For this review, take the finished solid that the model builds, in its own axes (mm). Face numbers are marked on the shaded views. A direction names the side the tool comes from. Coordinates: 2 decimals unless noted, no trailing zeros. Write each loop counter-clockwise with the first axis right and the second up, starting at its lowest first coordinate (ties: lowest second). Pieces come first, ordered by that corner, then holes.
```python
from build123d import *

# Parameters (mm, degrees)
BOSS_EXTRUDE1_DEPTH     = 15.748
BOSS_EXTRUDE3_DEPTH     = 47.752
SKETCH4_W               = 31.75
SKETCH4_H               = 47.752
BOSS_EXTRUDE4_DEPTH     = 15.748
FILLET1_R               = 12.7
CUT_EXTRUDE1_DEPTH      = 133.971969005
CUT_EXTRUDE1_DEPTH_BACK = 133.971969005
SKETCH5_R               = 9.525
CUT_EXTRUDE2_DEPTH      = 132.063135736
CUT_EXTRUDE2_DEPTH_BACK = 132.063135736
SKETCH6_R               = 9.525


with BuildPart() as part:
    # Sketch1 → Boss-Extrude1 (new body)
    with BuildSketch(Plane.XY):
        with BuildLine():
            Line((-28.575, 0), (-95.292827815, 0))
            Line((-95.292827815, 0), (-95.292827815, -79.502))
            Line((-95.292827815, -79.502), (95.207172185, -79.502))
            Line((95.207172185, -79.502), (95.207172185, 0))
            Line((95.207172185, 0), (28.575, 0))
            ThreePointArc((28.575, 0), (0, -28.575), (-28.575, 0))
        make_face()
    extrude(amount=BOSS_EXTRUDE1_DEPTH)

    # Sketch2 → Boss-Extrude3 (add)
    with BuildSketch(Plane.XY.offset(15.748)):
        with BuildLine():
            Line((-44.45, 0), (-44.45, -79.502))
            Line((-44.45, -79.502), (44.45, -79.502))
            Line((44.45, -79.502), (44.45, 0))
            Line((44.45, 0), (28.575, 0))
            ThreePointArc((28.575, 0), (0, -28.575), (-28.575, 0))
            Line((-28.575, 0), (-44.45, 0))
        make_face()
    extrude(amount=BOSS_EXTRUDE3_DEPTH)

    # Sketch4 → Boss-Extrude4 (add)
    with BuildSketch(Plane.XZ.offset(79.502)):
        with Locations((-60.325, 39.624)):
            Rectangle(SKETCH4_W, SKETCH4_H)
        with Locations((60.325, 39.624)):
            Rectangle(SKETCH4_W, SKETCH4_H)
    extrude(amount=-BOSS_EXTRUDE4_DEPTH)

    # Fillet1
    fillet1_edges = [part.edges().sort_by_distance(p)[0] for p in [
        (-76.2, -71.628, 63.5),
        (76.2, -71.628, 63.5),
    ]]
    fillet(fillet1_edges, radius=FILLET1_R)

    # Sketch5 → Cut-Extrude1 (cut, two sides: drawn at the far end of the back side and taken through both)
    with BuildSketch(Plane.XY.offset(15.748).offset(-CUT_EXTRUDE1_DEPTH_BACK)):
        with Locations((63.5, -28.702)):
            Circle(SKETCH5_R)
        with Locations((-63.5, -28.702)):
            Circle(SKETCH5_R)
    extrude(amount=CUT_EXTRUDE1_DEPTH + CUT_EXTRUDE1_DEPTH_BACK, mode=Mode.SUBTRACT)

    # Sketch6 → Cut-Extrude2 (cut, two sides: drawn at the far end of the back side and taken through both)
    with BuildSketch(Plane(origin=(0, -63.754, 0), x_dir=(1, 0, 0), z_dir=(0, 1, 0)).offset(-CUT_EXTRUDE2_DEPTH_BACK)):
        with Locations(Location((-58.42, -38.1, 0), (0, 0, 270))):
            Circle(SKETCH6_R)
        with Locations(Location((58.42, -38.1, 0), (0, 0, 270))):
            Circle(SKETCH6_R)
    extrude(amount=CUT_EXTRUDE2_DEPTH + CUT_EXTRUDE2_DEPTH_BACK, mode=Mode.SUBTRACT)


solid = part.part
```
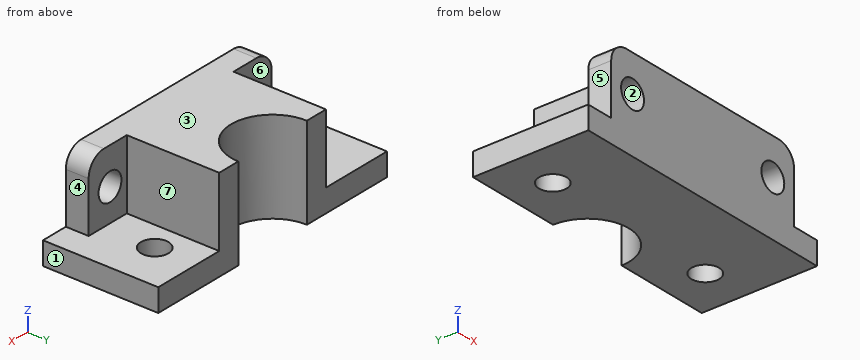
Q1. Add section A-A (z = 38.1). State the section outline as (x, y) points (3 decimals), then the cut area to 3 significant figures.
Ans:
outline: (-76.2, -79.502) - (-67.945, -79.502) - (-67.945, -63.754) - (-76.2, -63.754) - close; (-48.895, -79.502) - (48.895, -79.502) - (48.895, -63.754) - (44.45, -63.754) - (44.45, 0) - (28.575, 0) arc R28.575 cw to (-28.575, 0) - (-44.45, 0) - (-44.45, -63.754) - (-48.895, -63.754) - close; (67.945, -79.502) - (76.2, -79.502) - (76.2, -63.754) - (67.945, -63.754) - close
area: 6,190 mm2
Q2. Add section B-B (y = -67.5). State the section outline as (x, z) points (3 decimals).
Ans:
outline: (-95.293, 0) - (95.207, 0) - (95.207, 15.748) - (76.2, 15.748) - (76.2, 50.8) arc R12.7 ccw to (63.5, 63.5) - (-63.5, 63.5) arc R12.7 ccw to (-76.2, 50.8) - (-76.2, 15.748) - (-95.293, 15.748) - close; hole circle Ø19.05 at (-58.42, 38.1); hole circle Ø19.05 at (58.42, 38.1)
Q3. Draft analysis for pull direction X (two halves, no side actions). For the marked faces 1, 2 and 3, state which applies: +X half, -X half, draft (parallel to the pull), parting line (faces both ways), or undercut.
Ans:
face 1: +X half
face 2: undercut
face 3: draft
Q4. Add section C-C (y = -59). State the section outline as (x, z) points.
Ans:
outline: (-95.29, 0) - (95.21, 0) - (95.21, 15.75) - (44.45, 15.75) - (44.45, 63.5) - (-44.45, 63.5) - (-44.45, 15.75) - (-95.29, 15.75) - close
Q5. Tool access review of the marked faces 4, 5, 6 and 7: name each direction out of +Z, -Z, +X, -X, +Y, -Y from which nothing blocks a thin tool from reaching the whole face with its end or side.
Ans:
face 4: +Z, +X, +Y, -Y
face 5: +Z, -X, +Y, -Y
face 6: +Z, -X, +Y
face 7: +Z, +X, +Y
Q6. For probe 1 along X at (y, z) = (-75, 38); probe 2 along Y at (x, z) = (63.5, 6.5); probe 3 along Z at (x, y) = (-81.5, -49), list the stretches that pass through material, from the lowest coordinate up.
Ans:
probe 1: x = -76.2 to -67.94, -48.9 to 48.9, 67.94 to 76.2
probe 2: y = -79.5 to -38.23, -19.18 to 0
probe 3: z = 0 to 15.75
Q7. Add section D-D (x = 58.42). State the section outline as (y, z) points (3 decimals).
Ans:
outline: (-79.502, 0) - (-36.759, 0) - (-36.759, 15.748) - (-63.754, 15.748) - (-63.754, 28.575) - (-79.502, 28.575) - close; (-79.502, 47.625) - (-63.754, 47.625) - (-63.754, 63.5) - (-79.502, 63.5) - close; (-20.645, 0) - (0, 0) - (0, 15.748) - (-20.645, 15.748) - close
Q8. Clearance check with flat-ended pins moving along their axes: pin 1 Ø10 at (y, z) = (-12, 50.5) entering from -X; pin 2 Ø15.5 at (x, y) = (-67.5, -24) entering from +Z; pin 3 Ø16 at (x, z) = (57.5, 34) entering from +Y. State where each tip first meets the part, or that it passes through.
Ans:
pin 1: stops at x = -44.45
pin 2: stops at z = 15.75
pin 3: stops at y = -63.75
